Part model, mm, in its own coordinate system. Face numbers are marked on the shaded views. Give positions to 0.01 mm unless a question says otherwise; leave off trailing zeros. Write each loop counter-clockwise with the first axis right and the second up, starting at its lowest first coordinate (ties: lowest second). Pieces come first, ordered by that corner, then holes. Notation, with made-up numbers: M -31.5,-12 L -23.5,-12 A19 cw -23.5,25 Z; hole C 65.25,51 d7. An arc over 180 degrees is marked long. Use a Markdown table: item, result.
```python
from build123d import *

# Parameters (mm, degrees)
F0_W     = 62.741658
F0_H     = 10.648813
F1_DEPTH = 4.445
F2_R     = 3.967882
F3_DEPTH = 4.446
F4_R     = 5.08
F5_R     = 5.08


with BuildPart() as f1:
    # F0 (on Top) → F1 (new body)
    with BuildSketch(Plane.XY):
        with Locations((-14.9659, -2.158543)):
            Rectangle(F0_W, F0_H)
    extrude(amount=F1_DEPTH)

    # F2 (on face) → F3 (cut, through all)
    with BuildSketch(Plane.XY.offset(4.445)):
        with Locations((-34.9811, -2.158543)):
            Circle(F2_R)
        with Locations((5.0341, -2.158543)):
            Circle(F2_R)
        with Locations((-24.9735, -2.158543)):
            Circle(F2_R)
        with Locations((-14.9659, -2.158543)):
            Circle(F2_R)
        with Locations((-4.9659, -2.158543)):
            Circle(F2_R)
    extrude(amount=-F3_DEPTH, mode=Mode.SUBTRACT)

    # F4
    f4_edges = [f1.edges().sort_by_distance(p)[0] for p in [
        (-46.336729, 3.165863, 2.2225),
        (-46.336729, -7.48295, 2.2225),
    ]]
    fillet(f4_edges, radius=F4_R)

    # F5
    f5_edges = [f1.edges().sort_by_distance(p)[0] for p in [
        (16.404929, -7.48295, 2.2225),
        (16.404929, 3.165863, 2.2225),
    ]]
    fillet(f5_edges, radius=F5_R)


solid = f1.part
```
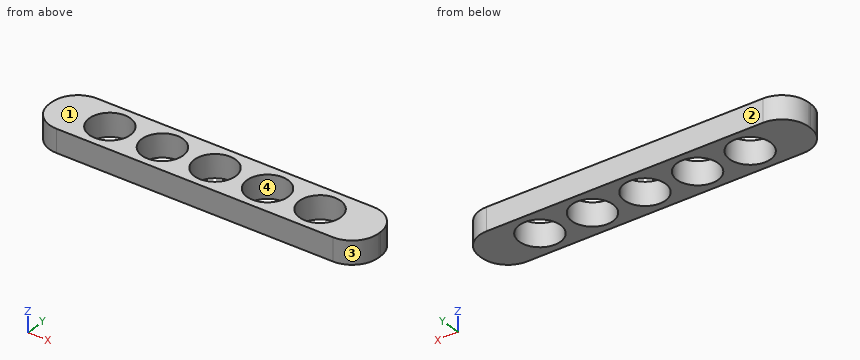
1. Cut at D-D, the plane y = 0.5. Give the cut face in (x, z) (3 decimals), then the cut area to 3 significant figures.
Findings below:
| item | result |
|---|---|
| outline | M -45.726,0 L -37.927,0 L -37.927,4.445 L -45.726,4.445 Z; M -32.036,0 L -27.919,0 L -27.919,4.445 L -32.036,4.445 Z; M -22.028,0 L -17.911,0 L -17.911,4.445 L -22.028,4.445 Z; M -12.02,0 L -7.911,0 L -7.911,4.445 L -12.02,4.445 Z; M -2.02,0 L 2.089,0 L 2.089,4.445 L -2.02,4.445 Z; M 7.98,0 L 15.795,0 L 15.795,4.445 L 7.98,4.445 Z |
| area | 143 mm2 |
2. Cut at C-C, the plane z = 1.05. Give the cut face in (x, y), then the cut area to 3 significant figures.
Findings below:
| item | result |
|---|---|
| outline | M -46.34,-2.4 A5.08 ccw -41.26,-7.48 L 11.32,-7.48 A5.08 ccw 16.4,-2.4 L 16.4,-1.91 A5.08 ccw 11.32,3.17 L -41.26,3.17 A5.08 ccw -46.34,-1.91 Z; hole C -34.98,-2.16 d7.94; hole C -24.97,-2.16 d7.94; hole C -14.97,-2.16 d7.94; hole C -4.97,-2.16 d7.94; hole C 5.03,-2.16 d7.94 |
| area | 399 mm2 |
3. Two-plate mould, pull along Y, no slides. Class the marked faces 1, 2, 3 and 4: released by +Y, released by -Y, zero draft, split by the parting line, or undercut.
Findings below:
| item | result |
|---|---|
| face 1 | zero draft |
| face 2 | released by +Y |
| face 3 | released by -Y |
| face 4 | undercut |
4. Drill centre lines: L1, parallel to X at y = -4.5, z = 3.5; L2, parallel to X at y = -2.75, z = 4.05; L3, parallel to Y at x = -37, z = 3.8. Where is each one in solid material? Low to high.
Findings below:
| item | result |
|---|---|
| L1 | -45.88 to -38.18, -31.78 to -28.18, -21.77 to -18.17, -11.76 to -8.17, -1.76 to 1.83, 8.24 to 15.95 |
| L2 | -46.32 to -38.9, -31.06 to -28.9, -21.05 to -18.89, -11.04 to -8.89, -1.04 to 1.11, 8.96 to 16.39 |
| L3 | -7.48 to -5.57, 1.26 to 3.17 |
5. Cut at A-A, the plane y = -5.25. Give the cut face in (x, z) (3 decimals), then the cut area to 3 significant figures.
Findings below:
| item | result |
|---|---|
| outline | M -45.464,0 L -37.468,0 L -37.468,4.445 L -45.464,4.445 Z; M -32.494,0 L -27.461,0 L -27.461,4.445 L -32.494,4.445 Z; M -22.486,0 L -17.453,0 L -17.453,4.445 L -22.486,4.445 Z; M -12.479,0 L -7.453,0 L -7.453,4.445 L -12.479,4.445 Z; M -2.479,0 L 2.547,0 L 2.547,4.445 L -2.479,4.445 Z; M 7.521,0 L 15.532,0 L 15.532,4.445 L 7.521,4.445 Z |
| area | 161 mm2 |
6. Drop flat-ended pins along their axis: P1, Ø2, axis at y = -5, z = 1.5, coming from the +X side; P2, Ø2, axis at y = -5, z = 3.5, coming from the -X side. Give the stop position or say it passes through.
Findings below:
| item | result |
|---|---|
| P1 | x = 16.15 |
| P2 | x = -46.08 |
7. Cut at B-B, the plane x = -17.5. Give the cut face in (y, z) (3 decimals), then the cut area to 3 significant figures.
Findings below:
| item | result |
|---|---|
| outline | M -7.483,0 L -5.212,0 L -5.212,4.445 L -7.483,4.445 Z; M 0.895,0 L 3.166,0 L 3.166,4.445 L 0.895,4.445 Z |
| area | 20.2 mm2 |
